Could you check a few things on this model? Use its own coordinates, in mm. Give positions to 0.01 mm unless a question says otherwise; leave off trailing zeros. Loops run counter-clockwise (first coordinate to the right, second up) from the corner with the lowest first, then second, coordinate; pieces in that order, holes last. Notation, with made-up numbers: (54, 46.25) - (73, 46.25) arc R31 cw to (73, 70.25) - close; hole circle Ø10 at (65, 37). An arc over 180 degrees is marked (long way). Answer in a Markdown table with one row per item. Add a question column.
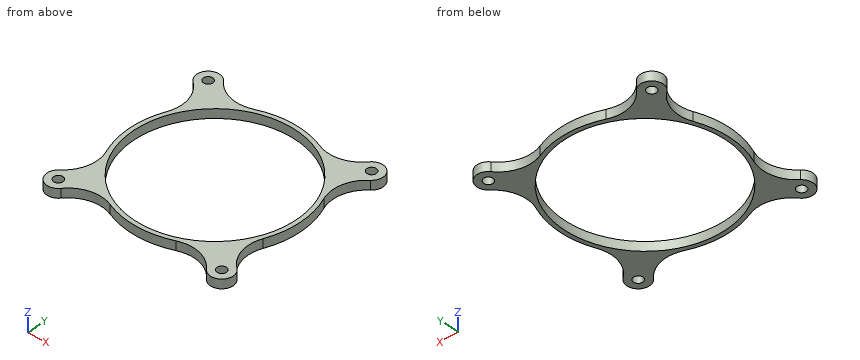
```python
from build123d import *

# Parameters (mm, degrees)
SKETCH2_R           = 34
SKETCH2_R_2         = 2.05
BOSS_EXTRUDE1_DEPTH = 4
CUT_EXTRUDE1_START  = -6
SKETCH3_R           = 35.75
SKETCH3_R_2         = 34
CUT_EXTRUDE1_DEPTH  = 10


with BuildPart() as part:
    # Sketch2 → Boss-Extrude1 (new body)
    with BuildSketch(Plane(origin=(0, 0, 0), x_dir=(0, 1, 0), z_dir=(0, 0, 1))):
        with BuildLine():
            ThreePointArc((-32.144333809, 39.168632909), (-39.597979746, 39.597979746), (-39.168632909, 32.144333809))
            ThreePointArc((-39.168632909, 32.144333809), (-33.957976607, 24.118514652), (-34.660047505, 14.575359582))
            ThreePointArc((-34.660047505, 14.575359582), (-37.6, 0), (-34.660047505, -14.575359582))
            ThreePointArc((-34.660047505, -14.575359582), (-33.957976607, -24.118514652), (-39.168632909, -32.144333809))
            ThreePointArc((-39.168632909, -32.144333809), (-39.597979746, -39.597979746), (-32.144333809, -39.168632909))
            ThreePointArc((-32.144333809, -39.168632909), (-24.118514652, -33.957976607), (-14.575359582, -34.660047505))
            ThreePointArc((-14.575359582, -34.660047505), (0, -37.6), (14.575359582, -34.660047505))
            ThreePointArc((14.575359582, -34.660047505), (24.118514652, -33.957976607), (32.144333809, -39.168632909))
            ThreePointArc((32.144333809, -39.168632909), (39.597979746, -39.597979746), (39.168632909, -32.144333809))
            ThreePointArc((39.168632909, -32.144333809), (33.957976607, -24.118514652), (34.660047505, -14.575359582))
            ThreePointArc((34.660047505, -14.575359582), (37.6, 0), (34.660047505, 14.575359582))
            ThreePointArc((34.660047505, 14.575359582), (33.957976607, 24.118514652), (39.168632909, 32.144333809))
            ThreePointArc((39.168632909, 32.144333809), (39.597979746, 39.597979746), (32.144333809, 39.168632909))
            ThreePointArc((32.144333809, 39.168632909), (24.118514652, 33.957976607), (14.575359582, 34.660047505))
            ThreePointArc((14.575359582, 34.660047505), (0, 37.6), (-14.575359582, 34.660047505))
            ThreePointArc((-14.575359582, 34.660047505), (-24.118514652, 33.957976607), (-32.144333809, 39.168632909))
        make_face()
        with Locations(Location((0, 0, 0), (0, 0, 270))):
            Circle(SKETCH2_R, mode=Mode.SUBTRACT)
        with Locations(Location((-36.062445841, 36.062445841, 0), (0, 0, 270))):
            Circle(SKETCH2_R_2, mode=Mode.SUBTRACT)
        with Locations(Location((36.062445841, 36.062445841, 0), (0, 0, 90))):
            Circle(SKETCH2_R_2, mode=Mode.SUBTRACT)
        with Locations(Location((36.062445841, -36.062445841, 0), (0, 0, 270))):
            Circle(SKETCH2_R_2, mode=Mode.SUBTRACT)
        with Locations(Location((-36.062445841, -36.062445841, 0), (0, 0, 90))):
            Circle(SKETCH2_R_2, mode=Mode.SUBTRACT)
    extrude(amount=BOSS_EXTRUDE1_DEPTH)

    # Sketch3 → Cut-Extrude1 (cut)
    with BuildSketch(Plane(origin=(0, 0, 0), x_dir=(0, 1, 0), z_dir=(0, 0, 1)).offset(CUT_EXTRUDE1_START)):
        with Locations(Location((0, 0, 0), (0, 0, 90))):
            Circle(SKETCH3_R)
        Circle(SKETCH3_R_2, mode=Mode.SUBTRACT)
    extrude(amount=CUT_EXTRUDE1_DEPTH, mode=Mode.SUBTRACT)


solid = part.part
```
(1) I want a section at A-A on x = 0. Please give me the cut outline in (y, z), then the cut area to 3 significant figures.
(2) For pin 1 Ø3.5 at (x, y) = (-36.06, 36.06) entering from +Z; pin 2 Ø2 at (y, z) = (14, 2) entering from -X, each with a flat end and sliding along its axis, tell me the tip position at first contact or that it passes through.
(3) Please list where these lines run through material, in increasing order: line 1 (Y direction, x = 33, z = 3); line 2 (Y direction, x = -16, z = 0.9); line 3 (X direction, y = -11.5, z = 0.3).
(4) I want a section at C-C on z = 1.55. Please give me the cut outline in (x, y), then the cut area to 3 significant figures.
Reported:
| question | item | result |
|---|---|---|
| 1 | outline | (-37.6, 0) - (-35.75, 0) - (-35.75, 4) - (-37.6, 4) - close; (35.75, 0) - (37.6, 0) - (37.6, 4) - (35.75, 4) - close |
| 1 | area | 14.8 mm² |
| 2 | pin 1 | through |
| 2 | pin 2 | x = -35.28 |
| 3 | line 1 | -40.01 to -13.75, 13.75 to 40.01 |
| 3 | line 2 | -34.14 to -31.97, 31.97 to 34.14 |
| 3 | line 3 | -35.8 to -33.85, 33.85 to 35.8 |
| 4 | outline | (-39.17, -32.14) arc R5 ccw (long way) to (-32.14, -39.17) arc R15 cw to (-14.58, -34.66) arc R37.6 ccw to (14.58, -34.66) arc R15 cw to (32.14, -39.17) arc R5 ccw (long way) to (39.17, -32.14) arc R15 cw to (34.66, -14.58) arc R37.6 ccw to (34.66, 14.58) arc R15 cw to (39.17, 32.14) arc R5 ccw (long way) to (32.14, 39.17) arc R15 cw to (14.58, 34.66) arc R37.6 ccw to (-14.58, 34.66) arc R15 cw to (-32.14, 39.17) arc R5 ccw (long way) to (-39.17, 32.14) arc R15 cw to (-34.66, 14.58) arc R37.6 ccw to (-34.66, -14.58) arc R15 cw to start; hole circle Ø4.1 at (-36.06, -36.06); hole circle Ø4.1 at (-36.06, 36.06); hole circle Ø71.5 at (0, 0); hole circle Ø4.1 at (36.06, -36.06); hole circle Ø4.1 at (36.06, 36.06) |
| 4 | area | 1,240 mm² |
